Source: three-view drawing plus pictorial views. Frame: mm from the lowest corner of the part. Give positions to 0.01 mm unless a question says otherwise; leave off trailing zeros. Loops run counter-clockwise (first coordinate to the right, second up) from the corner with the lowest first, then second, coordinate; pieces in that order, holes last. Notation, with made-up numbers: M -40,-18.75 L -16,-18.75 A30 ccw -16,3.25 Z; hole C 55.5,49.25 d9. An arc over 180 degrees is marked long. Answer as a JSON object with one key per item and string values. Group by question number.
1) Section query B-B on y = 6. Return loops of the section in (x, z), plus the area to 3 significant figures.
2) Section query C-C on z = 1.1. Return loops of the section in (x, y).
3) Section query A-A on x = 6. Return loops of the section in (y, z).
4) Ray query, L1, parallel to Y at x = 6, z = 1; L2, parallel to Y at x = 5.5, z = 0.7; L3, parallel to X at y = 3.5, z = 0.35 (1 decimal). Return the intervals inside material, ascending.
5) First-contact query: P1, Ø6, axis at x = 7, y = 7.5, coming from the -Z side; P2, Ø4.5, axis at x = 6, y = 6, coming from the -Z side. Flat tips, straight axial feed; report the tip coordinate or a pass-through.
6) Draft query along X for the marked faces 1, 2, 3 and 4. Return one class per face: +X half, -X half, draft (parallel to the pull), parting line (faces both ways), or undercut.
7) Section query D-D on x = 4. Return loops of the section in (y, z).
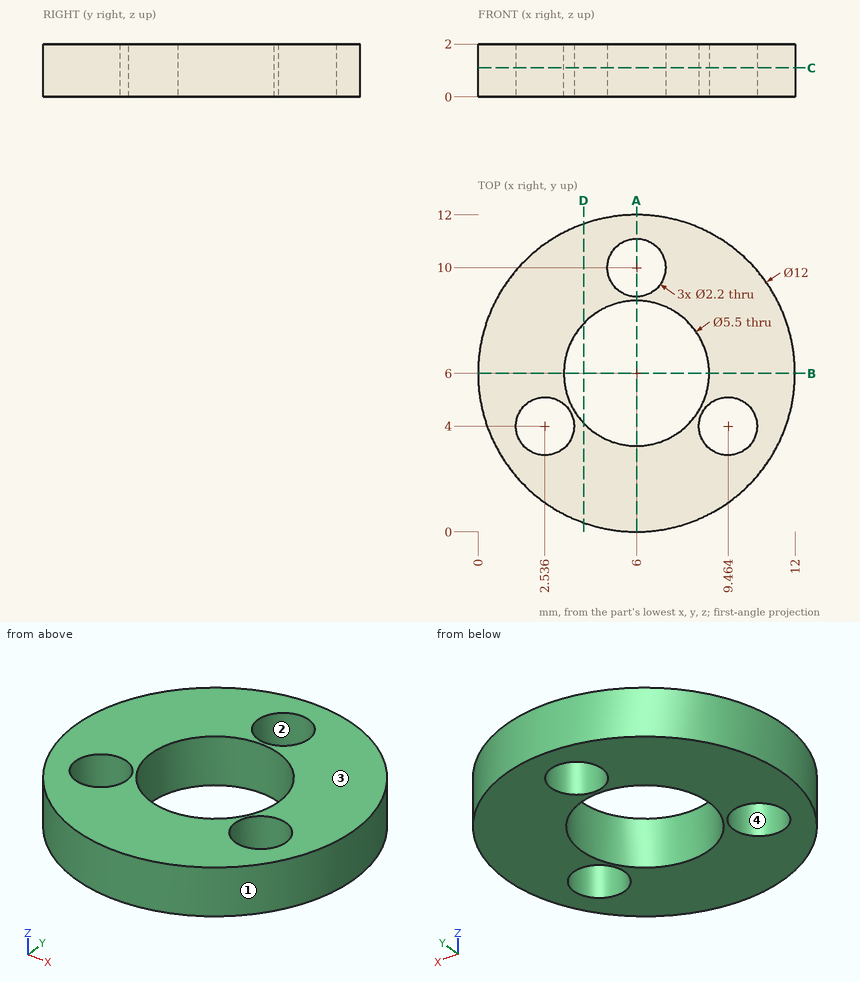
Output:
{
 "1": {"outline": "M 0,0 L 3.25,0 L 3.25,2 L 0,2 Z; M 8.75,0 L 12,0 L 12,2 L 8.75,2 Z", "area": "13.0 mm^2"},
 "2": {"outline": "C 6,6 d12; hole C 2.54,4 d2.2; hole C 6,6 d5.5; hole C 6,10 d2.2; hole C 9.46,4 d2.2"},
 "3": {"outline": "M 0,0 L 3.25,0 L 3.25,2 L 0,2 Z; M 8.75,0 L 8.9,0 L 8.9,2 L 8.75,2 Z; M 11.1,0 L 12,0 L 12,2 L 11.1,2 Z"},
 "4": {"L1": "y = 0 to 3.25, 8.75 to 8.9, 11.1 to 12", "L2": "y = 0.02 to 3.3, 8.7 to 9.02, 10.98 to 11.98", "L3": "x = 0.5 to 1.6, 3.5 to 4.9, 7.1 to 8.5, 10.4 to 11.5"},
 "5": {"P1": "stops at z = 0", "P2": "passes through"},
 "6": {"face 1": "parting line", "face 2": "undercut", "face 3": "draft", "face 4": "undercut"},
 "7": {"outline": "M 0.34,0 L 4.11,0 L 4.11,2 L 0.34,2 Z; M 7.89,0 L 11.66,0 L 11.66,2 L 7.89,2 Z"}
}
